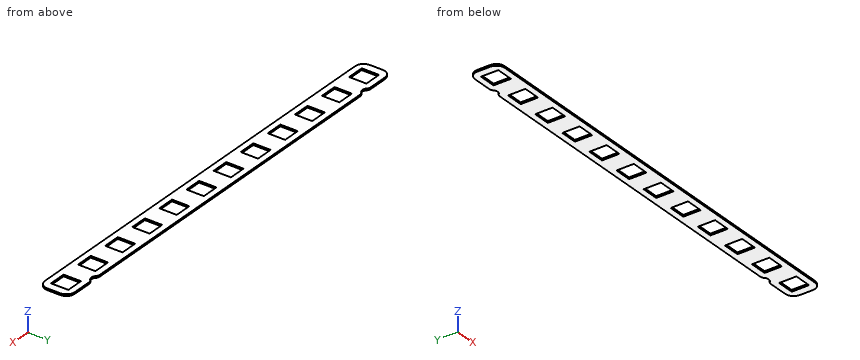
Autodesk Inventor part; units mm, degrees
ref_plane "YZ Plane" through (0, 0, 0) normal (1, 0, 0) x (0, 1, 0)
ref_plane "XZ Plane" through (0, 0, 0) normal (0, 1, 0) x (-1, 0, 0)
ref_plane "XY Plane" through (0, 0, 0) normal (0, 0, 1) x (1, 0, 0)
sketch "Skizze1" plane through (0, 0, 0) normal (0, 0, 1) x (1, 0, 0)
  line L0 (0, 0) -> (256, 0)
  line L1 (256, 0) -> (256, 17.5)
  line L2 (256, 17.5) -> (0, 17.5)
  line L3 (0, 17.5) -> (0, 0)
  line L4 (4.75, 3.65) -> (14.75, 3.65)
  line L5 (14.75, 3.65) -> (14.75, 13.85)
  line L6 (14.75, 13.85) -> (4.75, 13.85)
  line L7 (4.75, 13.85) -> (4.75, 3.65)
  line L8 (36.25, 3.65) -> (36.25, 13.85)
  line L9 (36.25, 13.85) -> (26.25, 13.85)
  line L10 (26.25, 13.85) -> (26.25, 3.65)
  line L11 (26.25, 3.65) -> (36.25, 3.65)
  line L12 (57.75, 3.65) -> (57.75, 13.85)
  line L13 (57.75, 13.85) -> (47.75, 13.85)
  line L14 (47.75, 13.85) -> (47.75, 3.65)
  line L15 (47.75, 3.65) -> (57.75, 3.65)
  line L16 (79.25, 3.65) -> (79.25, 13.85)
  line L17 (79.25, 13.85) -> (69.25, 13.85)
  line L18 (69.25, 13.85) -> (69.25, 3.65)
  line L19 (69.25, 3.65) -> (79.25, 3.65)
  line L20 (100.75, 3.65) -> (100.75, 13.85)
  line L21 (100.75, 13.85) -> (90.75, 13.85)
  line L22 (90.75, 13.85) -> (90.75, 3.65)
  line L23 (90.75, 3.65) -> (100.75, 3.65)
  line L24 (122.25, 3.65) -> (122.25, 13.85)
  line L25 (122.25, 13.85) -> (112.25, 13.85)
  line L26 (112.25, 13.85) -> (112.25, 3.65)
  line L27 (112.25, 3.65) -> (122.25, 3.65)
  line L28 (143.75, 3.65) -> (143.75, 13.85)
  line L29 (143.75, 13.85) -> (133.75, 13.85)
  line L30 (133.75, 13.85) -> (133.75, 3.65)
  line L31 (133.75, 3.65) -> (143.75, 3.65)
  line L32 (165.25, 3.65) -> (165.25, 13.85)
  line L33 (165.25, 13.85) -> (155.25, 13.85)
  line L34 (155.25, 13.85) -> (155.25, 3.65)
  line L35 (155.25, 3.65) -> (165.25, 3.65)
  line L36 (186.75, 3.65) -> (186.75, 13.85)
  line L37 (186.75, 13.85) -> (176.75, 13.85)
  line L38 (176.75, 13.85) -> (176.75, 3.65)
  line L39 (176.75, 3.65) -> (186.75, 3.65)
  line L40 (208.25, 3.65) -> (208.25, 13.85)
  line L41 (208.25, 13.85) -> (198.25, 13.85)
  line L42 (198.25, 13.85) -> (198.25, 3.65)
  line L43 (198.25, 3.65) -> (208.25, 3.65)
  line L44 (229.75, 3.65) -> (229.75, 13.85)
  line L45 (229.75, 13.85) -> (219.75, 13.85)
  line L46 (219.75, 13.85) -> (219.75, 3.65)
  line L47 (219.75, 3.65) -> (229.75, 3.65)
  line L48 (251.25, 3.65) -> (251.25, 13.85)
  line L49 (251.25, 13.85) -> (241.25, 13.85)
  line L50 (241.25, 13.85) -> (241.25, 3.65)
  line L51 (241.25, 3.65) -> (251.25, 3.65)
  arc A0 (232.7728, 17.5) -> (238.2272, 17.5) centre (235.5, 18.75) ccw
  arc A1 (17.7728, 17.5) -> (23.2272, 17.5) centre (20.5, 18.75) ccw
  point P0 (0, 8.75)
  point P1 (128, 17.5)
  point P2 (106.5, 8.75)
  point P3 (149.5, 8.75)
  point P4 (256, 8.75)
  point P5 (4.75, 8.75)
  point P6 (117.25, 3.65)
  point P7 (31.25, 3.65)
  point P8 (224.75, 3.65)
  point P9 (31.25, 13.85)
  point P10 (224.75, 13.85)
  dimension "d0" = 256
  dimension "d1" = 17.5
  dimension "d2" = 10.2
  dimension "d3" = 10
  dimension "d19" = 21.5
  dimension "d24" = 43
  dimension "d25" = 21.5
  dimension "d26" = 10.75
  dimension "d33" = 1.25
  dimension "d34" = 10.75
  dimension "d35" = 10.75
  dimension "d36" = 3
extrude "Extrusion1" add sketch "Skizze1" along normal blind 1 contours L3 L2 A1 A0 L1 L0
fillet "Rundung1" radius 5 4 edges at (256, 17.5, 0.5) (256, 0, 0.5) (0, 17.5, 0.5) (0, 0, 0.5)
fillet "Rundung2" radius 3 4 edges at (17.7728, 17.5, 0.5) (23.2272, 17.5, 0.5) (238.2272, 17.5, 0.5) (232.7728, 17.5, 0.5)
sketch "Skizze2" plane through (0, 0, 1) normal (0, 0, 1) x (1, 0, 0)
  arc A0 (0, 5) -> (5, 0) centre (5, 5) ccw
  line L0 (5, 0) -> (251, 0)
  arc A1 (251, 0) -> (256, 5) centre (251, 5) ccw
  line L1 (256, 5) -> (256, 12.5)
  arc A2 (256, 12.5) -> (251, 17.5) centre (251, 12.5) ccw
  line L2 (251, 17.5) -> (239.7353, 17.5)
  arc A3 (5, 17.5) -> (0, 12.5) centre (5, 12.5) ccw
  line L3 (0, 12.5) -> (0, 5)
  line L4 (251.25, 3.65) -> (241.25, 3.65)
  line L5 (241.25, 3.65) -> (241.25, 13.85)
  line L6 (241.25, 13.85) -> (251.25, 13.85)
  line L7 (251.25, 13.85) -> (251.25, 3.65)
  line L8 (229.75, 3.65) -> (219.75, 3.65)
  line L9 (219.75, 3.65) -> (219.75, 13.85)
  line L10 (219.75, 13.85) -> (229.75, 13.85)
  line L11 (229.75, 13.85) -> (229.75, 3.65)
  line L12 (208.25, 3.65) -> (198.25, 3.65)
  line L13 (198.25, 3.65) -> (198.25, 13.85)
  line L14 (198.25, 13.85) -> (208.25, 13.85)
  line L15 (208.25, 13.85) -> (208.25, 3.65)
  line L16 (186.75, 3.65) -> (176.75, 3.65)
  line L17 (176.75, 3.65) -> (176.75, 13.85)
  line L18 (176.75, 13.85) -> (186.75, 13.85)
  line L19 (186.75, 13.85) -> (186.75, 3.65)
  line L20 (165.25, 3.65) -> (155.25, 3.65)
  line L21 (155.25, 3.65) -> (155.25, 13.85)
  line L22 (155.25, 13.85) -> (165.25, 13.85)
  line L23 (165.25, 13.85) -> (165.25, 3.65)
  line L24 (143.75, 3.65) -> (133.75, 3.65)
  line L25 (133.75, 3.65) -> (133.75, 13.85)
  line L26 (133.75, 13.85) -> (143.75, 13.85)
  line L27 (143.75, 13.85) -> (143.75, 3.65)
  line L28 (122.25, 3.65) -> (112.25, 3.65)
  line L29 (112.25, 3.65) -> (112.25, 13.85)
  line L30 (112.25, 13.85) -> (122.25, 13.85)
  line L31 (122.25, 13.85) -> (122.25, 3.65)
  line L32 (100.75, 3.65) -> (90.75, 3.65)
  line L33 (90.75, 3.65) -> (90.75, 13.85)
  line L34 (90.75, 13.85) -> (100.75, 13.85)
  line L35 (100.75, 13.85) -> (100.75, 3.65)
  line L36 (79.25, 3.65) -> (69.25, 3.65)
  line L37 (69.25, 3.65) -> (69.25, 13.85)
  line L38 (69.25, 13.85) -> (79.25, 13.85)
  line L39 (79.25, 13.85) -> (79.25, 3.65)
  line L40 (57.75, 3.65) -> (47.75, 3.65)
  line L41 (47.75, 3.65) -> (47.75, 13.85)
  line L42 (47.75, 13.85) -> (57.75, 13.85)
  line L43 (57.75, 13.85) -> (57.75, 3.65)
  line L44 (36.25, 3.65) -> (26.25, 3.65)
  line L45 (26.25, 3.65) -> (26.25, 13.85)
  line L46 (26.25, 13.85) -> (36.25, 13.85)
  line L47 (36.25, 13.85) -> (36.25, 3.65)
  line L48 (4.75, 3.65) -> (4.75, 13.85)
  line L49 (4.75, 13.85) -> (14.75, 13.85)
  line L50 (14.75, 13.85) -> (14.75, 3.65)
  line L51 (14.75, 3.65) -> (4.75, 3.65)
  arc A4 (233.3824, 16.625) -> (237.6176, 16.625) centre (235.5, 18.75) ccw
  line L52 (231.2647, 17.5) -> (24.7353, 17.5)
  arc A5 (18.3824, 16.625) -> (22.6176, 16.625) centre (20.5, 18.75) ccw
  line L53 (16.2647, 17.5) -> (5, 17.5)
  arc A6 (233.3824, 16.625) -> (231.2647, 17.5) centre (231.2647, 14.5) ccw
  arc A7 (24.7353, 17.5) -> (22.6176, 16.625) centre (24.7353, 14.5) ccw
  arc A8 (18.3824, 16.625) -> (16.2647, 17.5) centre (16.2647, 14.5) ccw
  arc A9 (239.7353, 17.5) -> (237.6176, 16.625) centre (239.7353, 14.5) ccw
  point P0 (0, 0)
equation "\"Biegeradius\" = Stärke"
equation "\"BreiteBiegungsfreistellung\" = Stärke"
equation "\"TiefeBiegungsfreistellung\" = 0.5 * Stärke"
equation "\"GrößeEckenfreistellung\" = 4 * Stärke"
equation "\"MinimalRest\" = 2 * Stärke"
equation "\"Übergangsradius\" = Biegeradius"
equation "\"JacobiRadiusGröße\" = Biegeradius"
equation "\"Abstandsgröße\" = Stärke"
properties part number "bat_contacts_v2_plate_long" material "Kupfer"
For this review, take the finished solid that the model builds, in its own axes (mm). Round coordinates to 2 decimals unless told otherwise and drop trailing zeros. Loops run counter-clockwise (first coordinate to the right, second up) from the corner with the lowest first, then second, coordinate; pieces in that order, holes last. Notation, with made-up numbers: (-20, 69) - (-5, 69) arc R5 ccw to (-5, 76) - close; hole circle Ø6 at (-19.75, 58). An arc over 180 degrees is marked (long way). Use one line per item in the form item = value.
1) We need section A-A on x = 141. Write out the cut boundary in (y, z), then the cut area to 3 significant figures.
Solutions:
outline = (0, 0) - (3.65, 0) - (3.65, 1) - (0, 1) - close; (13.85, 0) - (17.5, 0) - (17.5, 1) - (13.85, 1) - close
area = 7.30 mm2
2) We need section B-B on y = 9.5. State how many separate pieces and enclosed holes the cut face has, then the cut area to 3 significant figures.
Solutions:
separate_pieces = 13
enclosed_holes = 0
area = 136 mm2
3) Wall thickness on probe 1 along Y at (x, z) = (164.5, 0.1); probe 2 along Y at (x, z) = (19, 0.7); probe 3 along X at (y, z) = (1.5, 0.4): over which ranges is each line inside the solid? List them lowest first.
Solutions:
probe_1 = 0 to 3.65, 13.85 to 17.5
probe_2 = 0 to 16.15
probe_3 = 1.43 to 254.57
